Autodesk Inventor part; units mm, degrees
ref_plane "YZ Plane" through (0, 0, 0) normal (1, 0, 0) x (0, 1, 0)
ref_plane "XZ Plane" through (0, 0, 0) normal (0, 1, 0) x (-1, 0, 0)
ref_plane "XY Plane" through (0, 0, 0) normal (0, 0, 1) x (1, 0, 0)
sketch "Sketch2" plane through (0, 0, 0) normal (0, 1, 0) x (-1, 0, 0)
  line L0 (0, -0.1) -> (0, 1.3)
  line L1 (-4.8, 0) -> (3.6, 0)
  line L2 (-0.5, 0) -> (0.5, 0)
  line L3 (0.5, 0) -> (0.5, 1)
  line L4 (0.5, 1) -> (-0.5, 1)
  line L5 (-0.5, 1) -> (-0.5, 0)
  line L6 (2, 0) -> (3, 0)
  line L7 (3, 0) -> (3, 1)
  line L8 (3, 1) -> (2, 1)
  line L9 (2, 1) -> (2, 0)
  line L10 (-2, 0) -> (-3, 0)
  line L11 (-3, 0) -> (-3, 1)
  line L12 (-3, 1) -> (-2, 1)
  line L13 (-2, 1) -> (-2, 0)
  dimension "d0" = 6
  dimension "d1" = 1
  dimension "d2" = 1
extrude "Extrusion1" add sketch "Sketch2" along normal mid plane 0.5
sketch "Sketch3" plane through (0, 0, 0) normal (0, 1, 0) x (-1, 0, 0)
  line L0 (0, -1.18) -> (0, 15.34)
  line L1 (-0.5, 1) -> (0.5, 1)
  line L2 (-3.5, 8.8) -> (3.5, 8.8)
  line L3 (3.5, 8.8) -> (3.5, 0.8)
  line L4 (3.5, 0.8) -> (-3.5, 0.8)
  line L5 (-3.5, 0.8) -> (-3.5, 8.8)
  point P0 (0, 0)
  dimension "d5" = 0.2
  dimension "d6" = 8
  dimension "d7" = 7
extrude "Extrusion2" add sketch "Sketch3" along normal mid plane 2
draft "FaceDraft1" angle 5 pull direction (0, -1, 0) faces at (3.5, 0.3333, 6.1333) (-0.1667, 0.75, 0.8) (-3.5, -0.3333, 6.1333) (-1.1667, 0.3333, 8.8) fixed edges at (3.5, -1, 4.8) (0, -1, 0.8) (-3.5, -1, 4.8) (0, -1, 8.8)
properties part number "config - chip stand"
Work out the finished part from the listing and answer in its coordinate system (mm). Give positions to 0.01 mm unless a question says otherwise; leave off trailing zeros. Loops run counter-clockwise (first coordinate to the right, second up) from the corner with the lowest first, then second, coordinate; pieces in that order, holes last. Notation, with made-up numbers: (18.5, 50.25) -> (53.5, 50.25) arc R3 ccw to (53.5, 54.25) -> close; hole circle Ø5 at (40, -5.5). An arc over 180 degrees is marked (long way). Use a Markdown table: item, result. Add a question column.
1. Section B-B on x = 2.25 is taken. Determine the outline of the cut face in (y, z), and give its area (3 significant figures).
2. Determine the mould class of faces 1 (the flat face through (0, 1, 5)), 2 (the flat face through (0.051, -0.014, 8.886)), 3 (the flat face through (-0.051, -0.458, 0.753)) for opening direction Y: released by +Y, released by -Y, zero draft, split by the parting line, or undercut.
3. Find the intervals of material crossed by probe 1 along Z at (x, y) = (-0.75, 0.3); probe 2 along X at (y, z) = (0.1, 4.5); probe 3 along Z at (x, y) = (2.5, 0.95), in increasing order.
4. Section A-A on z = 0.5 is taken. Determine the outline of the cut face in (x, y), and give its area (3 significant figures).
5. Section C-C on z = 7.5 is taken. Determine the outline of the cut face in (x, y).
6. Section D-D on y = 0.7 is taken. Determine the outline of the cut face in (x, z).
Results below:
| question | item | result |
|---|---|---|
| 1 | outline | (-1, 0.8) -> (-0.25, 0.73) -> (-0.25, 0) -> (0.25, 0) -> (0.25, 0.69) -> (1, 0.63) -> (1, 8.97) -> (-1, 8.8) -> close |
| 1 | area | 16.7 mm^2 |
| 2 | face 1 | released by +Y |
| 2 | face 2 | released by -Y |
| 2 | face 3 | undercut |
| 3 | probe 1 | z = 0.69 to 8.91 |
| 3 | probe 2 | x = -3.6 to 3.6 |
| 3 | probe 3 | z = 0.63 to 8.97 |
| 4 | outline | (-3, -0.25) -> (-2, -0.25) -> (-2, 0.25) -> (-3, 0.25) -> close; (-0.5, -0.25) -> (0.5, -0.25) -> (0.5, 0.25) -> (-0.5, 0.25) -> close; (2, -0.25) -> (3, -0.25) -> (3, 0.25) -> (2, 0.25) -> close |
| 4 | area | 1.50 mm^2 |
| 5 | outline | (-3.67, 1) -> (-3.5, -1) -> (3.5, -1) -> (3.67, 1) -> close |
| 6 | outline | (-3.65, 0.65) -> (3.65, 0.65) -> (3.65, 8.95) -> (-3.65, 8.95) -> close |
